The model under review builds one solid part; all positions refer to its coordinate system, in mm. Face numbers are marked on the shaded views. A direction names the side the tool comes from. Give positions to 0.01 mm unless a question says otherwise; leave off trailing zeros. Loops run counter-clockwise (first coordinate to the right, second up) from the corner with the lowest first, then second, coordinate; pieces in that order, holes last. Notation, with made-up numbers: M 41.25,72.25 L 96.25,72.25 A22 ccw 96.25,87.25 Z; hole C 29.5,69 d8. An arc over 180 degrees is marked long. Put each result on its own line as item: value. Start each with the question number.
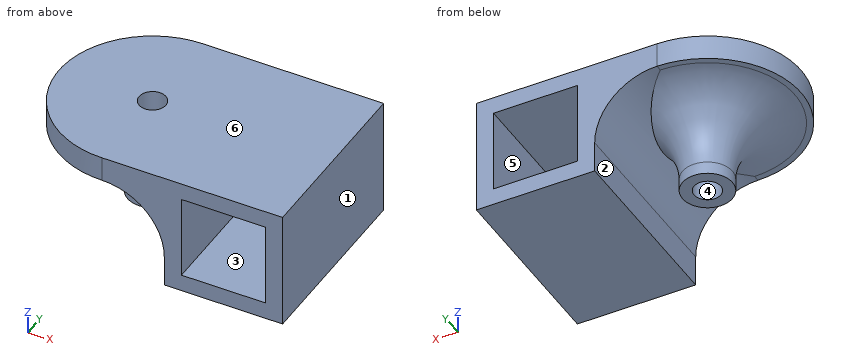
```python
from build123d import *
from build123d import SkipClean  # not in build123d's __all__

# Parameters (mm, degrees)
F0_W         = 19
F0_H         = 19
F0_W_2       = 13.5
F0_H_2       = 13.5
F1_DEPTH     = 15
F2_R         = 4
F2_R_2       = 2.15
F3_DEPTH     = 4
F4_DEPTH     = 16
F5_T9_DEPTH  = 30
F5_S10_R     = 2.15
F5_T11_DEPTH = 18


# Not quite as in the source:
# - a fillet or chamfer that OpenCascade refuses, or shapes differently, is made with other operations: its cross-section is extruded or revolved along the edge and cut away or added


with BuildPart() as f1:
    # F0 (on Front) → F1 (new body, symmetric)
    with BuildSketch(Plane.XZ):
        Rectangle(F0_W, F0_H)
        Rectangle(F0_W_2, F0_H_2, mode=Mode.SUBTRACT)
    extrude(amount=F1_DEPTH, both=True)

    # F2 (on face) → F3 (join)
    with BuildSketch(Plane.XY.offset(9.5)):
        with BuildLine():
            Line((-9.5, -15), (-9.5, 15))
            Line((-9.5, 15), (-19.5, 15))
            ThreePointArc((-19.5, 15), (-34.5, 0), (-19.5, -15))
            Line((-19.5, -15), (-9.5, -15))
        make_face()
        with Locations((-19.5, 0)):
            Circle(F2_R, mode=Mode.SUBTRACT)
        with Locations((-19.5, 0)):
            Circle(F2_R)
        with Locations((-19.5, 0)):
            Circle(F2_R_2, mode=Mode.SUBTRACT)
    extrude(amount=-F3_DEPTH)

    # F2 (on face) → F4 (join)
    with BuildSketch(Plane.XY.offset(9.5)):
        with Locations((-19.5, 0)):
            Circle(F2_R)
        with Locations((-19.5, 0)):
            Circle(F2_R_2, mode=Mode.SUBTRACT)
    extrude(amount=-F4_DEPTH)

    # F5: fillet of radius 10 on 2 edges, made by hand


with BuildPart() as f5_tool2:
    # F5_s3 → F5_t4 (revolve)
    with BuildSketch(Plane.XZ):
        with BuildLine():
            ThreePointArc((-5.5, 5.5), (-12.5710678119, 2.5710678119), (-15.5, -4.5))
            Line((-15.5, -4.5), (-15.5, 5.5))
            Line((-15.5, 5.5), (-5.5, 5.5))
        make_face()
    revolve(axis=Axis((-19.5, 0, 5.5), (0, 0, 1)))

    split(bisect_by=Plane.YZ.offset(-6.75), keep=Keep.BOTTOM)


with BuildPart() as f1_1:
    add(f1.part, clean=False)

    # F5_t1: union F5_tool2
    add(f5_tool2.part)


with BuildPart() as f5_tool7:
    # F5_s8 → F5_t9 (new body)
    with BuildSketch(Plane.XZ.offset(15)):
        with BuildLine():
            ThreePointArc((-9.5, -4.5), (-12.4289321881, 2.5710678119), (-19.5, 5.5))
            Line((-19.5, 5.5), (-9.5, 5.5))
            Line((-9.5, 5.5), (-9.5, -4.5))
        make_face()
    extrude(amount=-F5_T9_DEPTH)

    # F5_s10 → F5_t11 (cut, symmetric)
    with BuildSketch(Plane.XY.offset(0.5)):
        with Locations((-19.5, 0)):
            Circle(F5_S10_R)
    with SkipClean():  # cleaning this boolean's faces spoils the solid; the shape is the same uncleaned
        extrude(amount=F5_T11_DEPTH, both=True, mode=Mode.SUBTRACT)


with BuildPart() as f1_2:
    add(f1_1.part, clean=False)

    # F5_t6: union F5_tool7
    add(f5_tool7.part)


solid = f1_2.part
```
Item 1: Draft analysis for pull direction Z (two halves, no side actions). For the marked faces 4, 5 and 6, state which applies: +Z half, -Z half, draft (parallel to the pull), parting line (faces both ways), or undercut.
Item 2: Consider section A-A, the plane z = -6. Write out the cut boundary in (x, y).
Item 3: To check wall thickness, follow L1, parallel to Y at x = -19.5, z = 6.25; L2, parallel to X at y = 3.5, z = -1; L3, parallel to Z at x = -4.5, y = -1.5. State the ranges of each line that lie inside material, in increasing order. Write a range as [from, to].
Item 4: Clearance check with flat-ended pins moving along their axes: pin 1 Ø4 at (y, z) = (3, 0) entering from -X; pin 2 Ø3 at (x, z) = (-22, 6.5) entering from -Y; pin 3 Ø7.5 at (x, y) = (-28.5, -0.5) entering from -Z; pin 4 Ø2.5 at (x, y) = (-19.5, 0) entering from -Z. State where each tip first meets the part, or that it passes through.
Item 5: Consider section B-B, the plane x = -1. Write out the cut boundary in (y, z), plus the area to 3 significant figures.
Item 6: Tool access review of the marked faces 1, 2 and 3: name each direction out of +Z, -Z, +X, -X, +Y, -Y from which nothing blocks a thin tool from reaching the whole face with its end or side.
Item 7: Consider section C-C, the plane y = 0. Write out the cut boundary in (x, z).
Item 8: Consider section D-D, the plane z = -1.25. Write out the cut boundary in (x, y), plus the area to 3 significant figures.
Report:
1. face 4: draft
1. face 5: undercut
1. face 6: +Z half
2. outline: C -19.5,0 d8; M -9.5,-15 L -6.75,-15 L -6.75,15 L -9.5,15 Z; M 6.75,-15 L 9.5,-15 L 9.5,15 L 6.75,15 Z; hole C -19.5,0 d4.3
3. L1: [-15, -2.15], [2.15, 15]
3. L2: [-22.53, -16.47], [-10.13, -6.75], [6.75, 9.5]
3. L3: [-9.5, -6.75], [6.75, 9.5]
4. pin 1: x = -25.36
4. pin 2: y = -14.97
4. pin 3: z = 0.37
4. pin 4: through
5. outline: M -15,-9.5 L 15,-9.5 L 15,-6.75 L -15,-6.75 Z; M -15,6.75 L 15,6.75 L 15,9.5 L -15,9.5 Z
5. area: 165 mm²
6. face 1: +Z, -Z, +X, +Y, -Y
6. face 2: -Z, +Y, -Y
6. face 3: +Y, -Y
7. outline: M -34.5,5.5 L -33.5,5.5 A10 cw -23.5,-4.5 L -23.5,-6.5 L -21.65,-6.5 L -21.65,9.5 L -34.5,9.5 Z; M -17.35,-6.5 L -15.5,-6.5 L -15.5,-4.5 A10 cw -12.5,2.64 A10 cw -9.5,-4.5 L -9.5,-9.5 L 9.5,-9.5 L 9.5,9.5 L -17.35,9.5 Z; hole M -6.75,-6.75 L 6.75,-6.75 L 6.75,6.75 L -6.75,6.75 Z
8. outline: C -19.5,0 d9.09; M -10.04,-15 L -6.75,-15 L -6.75,15 L -10.04,15 Z; M 6.75,-15 L 9.5,-15 L 9.5,15 L 6.75,15 Z; hole C -19.5,0 d4.3
8. area: 232 mm²
